Build history of the part. All positions in model axes, mm. Face numbers are marked on the shaded views. A direction names the side the tool comes from. Give positions to 0.01 mm unless a question says otherwise; leave off trailing zeros. Loops run counter-clockwise (first coordinate to the right, second up) from the corner with the lowest first, then second, coordinate; pieces in that order, holes last. Notation, with made-up numbers: (10, 55) -> (43, 55) arc R12 cw to (43, 77) -> close; hole circle Ø8 at (26.25, -25.5). An arc over 180 degrees is marked (long way). One line per question, with ' | ' between items. Start each with the question number.
(1) Slice it at B-B, the plane y = 66. Write the cut outline in (x, z), then the cut area to 3 significant figures.
(2) Drill centre lines: L1, parallel to X at y = 3, z = -111; L2, parallel to Y at x = 41.5, z = -127.5; L3, parallel to Z at x = 137, y = 49. Where is each one in solid material? Low to high. Write a range as from..to.
(3) Slice it at A-A, the plane z = -102.5. Write the cut outline in (x, y), then the cut area to 3 significant figures.
(4) Flat gauge pins, fed straight in: pin 1 Ø3 at (x, z) = (111.5, 69) entering from +Y; pin 2 Ø1 at (x, y) = (-135.5, 20.5) entering from +Z. Where does each tip first touch, or does it go through?
(5) 3-axis set-ups, long thin cutter, end or side, ignore diameter. For the marked faces 5 and 6: which of +Z, -Z, +X, -X, +Y, -Y reach the whole face in a straight line?
(6) Slice it at C-C, the plane x = 42.5. Write the cut outline in (y, z), then the cut area to 3 significant figures.
(7) Mould opens along X. For the marked faces 1, 2, 3 and 4 say: pulls with the +X half, pulls with the -X half, needs draft (parallel to the pull), parting line crosses it, or undercut.
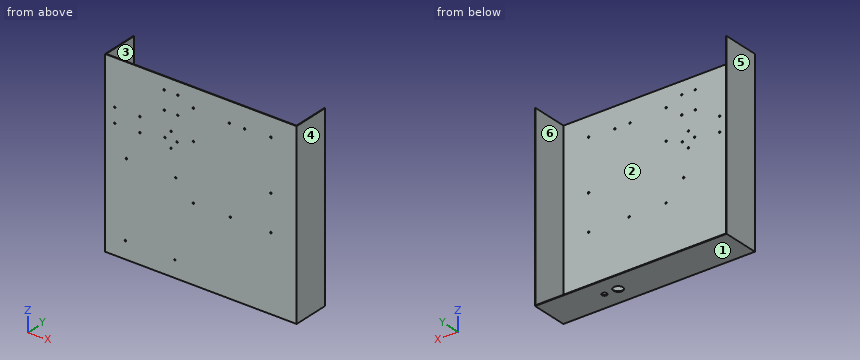
```python
from build123d import *

# Parameters (mm, degrees)
SKETCH1_W           = 431.8
SKETCH1_H           = 406.4
BOSS_EXTRUDE1_DEPTH = 82.55
SHELL1_T            = -1.4351
SKETCH2_W           = 431.8
SKETCH2_H           = 82.55
CUT_EXTRUDE1_DEPTH  = 1.5875
SKETCH4_R           = 1.63195
CUT_EXTRUDE3_DEPTH  = 160.02
SKETCH8_R           = 10.668
SKETCH8_R_2         = 5.715
CUT_EXTRUDE7_DEPTH  = 405.8125
SKETCH9_R           = 1.63195
SKETCH9_R_2         = 1.7145
CUT_EXTRUDE8_DEPTH  = 2.54
SKETCH3_R           = 1.75
CUT_EXTRUDE2_DEPTH  = 160.02
SKETCH5_R           = 1.63195
CUT_EXTRUDE6_DEPTH  = 2.4351


with BuildPart() as part:
    # Sketch1 → Boss-Extrude1 (new body)
    with BuildSketch(Plane(origin=(0, 0, 0), x_dir=(1, 0, 0), z_dir=(0, 1, 0))):
        Rectangle(SKETCH1_W, SKETCH1_H)
    extrude(amount=BOSS_EXTRUDE1_DEPTH)

    # Shell1
    shell1_openings = [part.faces().sort_by_distance(p)[0] for p in [
        (0, 82.55, 0),
    ]]
    offset(amount=SHELL1_T, openings=shell1_openings, kind=Kind.INTERSECTION)

    # Sketch2 → Cut-Extrude1 (cut)
    with BuildSketch(Plane.XY.offset(203.2)):
        with Locations((0, 41.275)):
            Rectangle(SKETCH2_W, SKETCH2_H)
    extrude(amount=-CUT_EXTRUDE1_DEPTH, mode=Mode.SUBTRACT)

    # Sketch4 → Cut-Extrude3 (cut)
    with BuildSketch(Plane(origin=(0, 1.4351, 0), x_dir=(1, 0, 0), z_dir=(0, 1, 0))):
        with Locations((-170.0149, 164.665635276)):
            Circle(SKETCH4_R)
        with Locations((-58.517028555, 166.012000494)):
            Circle(SKETCH4_R)
        with Locations((-167.978484272, -3.978070052)):
            Circle(SKETCH4_R)
        with Locations((-56.480612827, -2.631704835)):
            Circle(SKETCH4_R)
    extrude(amount=-CUT_EXTRUDE3_DEPTH, mode=Mode.SUBTRACT)

    # Sketch8 → Cut-Extrude7 (cut, through all)
    with BuildSketch(Plane(origin=(0, 0, -203.2), x_dir=(-1, 0, 0), z_dir=(0, 0, -1))):
        with Locations((-60.463632171, 41.275)):
            Circle(SKETCH8_R)
        with Locations((-91.444997416, 41.275)):
            Circle(SKETCH8_R_2)
    extrude(amount=-CUT_EXTRUDE7_DEPTH, mode=Mode.SUBTRACT)

    # Sketch9 → Cut-Extrude8 (cut)
    with BuildSketch(Plane(origin=(0, 1.4351, 0), x_dir=(1, 0, 0), z_dir=(0, 1, 0))):
        with Locations((-52.00702029, -132.161335594)):
            Circle(SKETCH9_R)
        with Locations((-52.00702029, -173.518885594)):
            Circle(SKETCH9_R)
        with Locations((-82.52512029, -173.518885594)):
            Circle(SKETCH9_R)
        with Locations((-82.52512029, -132.161335594)):
            Circle(SKETCH9_R_2)
        with Locations((-137.473717268, -100.235094157)):
            Circle(SKETCH9_R)
        with Locations((-194.242717268, -100.235094157)):
            Circle(SKETCH9_R)
        with Locations((-137.473717268, -67.430994157)):
            Circle(SKETCH9_R)
        with Locations((-194.242717268, -67.430994157)):
            Circle(SKETCH9_R)
    extrude(amount=-CUT_EXTRUDE8_DEPTH, mode=Mode.SUBTRACT)

    # Sketch3 → Cut-Extrude2 (cut)
    with BuildSketch(Plane(origin=(0, 1.4351, 0), x_dir=(1, 0, 0), z_dir=(0, 1, 0))):
        with Locations((157.934614453, 35.850005932)):
            Circle(SKETCH3_R)
        with Locations((157.934614453, -44.649994068)):
            Circle(SKETCH3_R)
        with Locations((157.934614453, -158.899994068)):
            Circle(SKETCH3_R)
        with Locations((98.434614453, -155.649994068)):
            Circle(SKETCH3_R)
        with Locations((64.444614453, -155.649994068)):
            Circle(SKETCH3_R)
        with Locations((-16.815385547, -158.899994068)):
            Circle(SKETCH3_R)
        with Locations((66.434614453, 35.850005932)):
            Circle(SKETCH3_R)
        with Locations((-16.815385547, 35.850005932)):
            Circle(SKETCH3_R)
        with Locations((-16.815385547, -90.649994068)):
            Circle(SKETCH3_R)
    extrude(amount=-CUT_EXTRUDE2_DEPTH, mode=Mode.SUBTRACT)

    # Sketch5 → Cut-Extrude6 (cut, through all)
    with BuildSketch(Plane(origin=(0, 1.4351, 0), x_dir=(1, 0, 0), z_dir=(0, 1, 0))):
        with Locations((-67.248855215, -59.585919699)):
            Circle(SKETCH5_R)
        with Locations((-67.248855215, -94.129919699)):
            Circle(SKETCH5_R)
        with Locations((-80.964855215, -76.857919699)):
            Circle(SKETCH5_R)
        with Locations((-53.532855215, -76.857919699)):
            Circle(SKETCH5_R)
    extrude(amount=-CUT_EXTRUDE6_DEPTH, mode=Mode.SUBTRACT)


solid = part.part
```
Final values:
1) outline: (-215.9, -203.2) -> (215.9, -203.2) -> (215.9, 201.61) -> (214.46, 201.61) -> (214.46, -201.76) -> (-214.46, -201.76) -> (-214.46, 201.61) -> (-215.9, 201.61) -> close | area: 1,780 mm2
2) L1: -215.9..-214.46, 214.46..215.9 | L2: 0..1.44 | L3: -203.2..-201.76
3) outline: (-215.9, 0) -> (215.9, 0) -> (215.9, 82.55) -> (214.46, 82.55) -> (214.46, 1.44) -> (-214.46, 1.44) -> (-214.46, 82.55) -> (-215.9, 82.55) -> close | area: 852 mm2
4) pin 1: y = 1.44 | pin 2: z = -201.76
5) face 5: +Z, -Z, -X, +Y, -Y | face 6: +Z, +Y
6) outline: (0, -203.2) -> (82.55, -203.2) -> (82.55, -201.76) -> (1.44, -201.76) -> (1.44, 201.61) -> (0, 201.61) -> close | area: 697 mm2
7) face 1: needs draft | face 2: undercut | face 3: undercut | face 4: pulls with the +X half
